```python
from build123d import *

# Parameters (mm, degrees)
F0_W     = 9.525
F0_H     = 18.034
F0_R     = 2.159
F1_DEPTH = 3.175


with BuildPart() as f1:
    # F0 (on Top) → F1 (new body)
    with BuildSketch(Plane.XY):
        with Locations((4.7625, -9.017)):
            Rectangle(F0_W, F0_H)
        with Locations((4.7625, -2.54)):
            Circle(F0_R, mode=Mode.SUBTRACT)
        Polygon((0, -18.034), (0, 0), (-2.54, 0), (-2.54, -21.59), (0, -21.59), align=None)
        Polygon((12.065, 0), (9.525, 0), (9.525, -18.034), (9.525, -21.59), (12.065, -21.59), align=None)
        Polygon((-2.54, 0), (0, 0), (9.525, 0), (12.065, 0), (12.065, 2.54), (-2.54, 2.54), align=None)
        Polygon((9.525, -21.59), (0, -21.59), (-2.54, -21.59), (-2.54, -24.13), (12.065, -24.13), (12.065, -21.59), align=None)
    extrude(amount=F1_DEPTH)


solid = f1.part
```
Geometry check sheet. Reference: the model listing, model coordinates, mm. A direction names the side the tool comes from. Give positions to 0.01 mm unless a question says otherwise; leave off trailing zeros. Order: outer loops, then holes, each group sorted by start corner. A loop starts at its lowest first (then second) coordinate and runs counter-clockwise, first axis right, second up.
1. Section check C-C, the plane z = 1.95. Enter the section's corners in (x, y) (1 decimal).
2. Section check B-B, the plane y = -2.54. Enter the section's corners in (x, z) (1 decimal).
3. Section check A-A, the plane x = 0.75. Enter the section's corners in (y, z) (3 decimals), and give its area (3 significant figures).
4. Thickness scan on L1, parallel to Y at x = 0.25, z = 3; L2, parallel to Y at x = 4.5, z = 0.4; L3, parallel to X at y = -21.5, z = 0.3 (3 decimals). Record the ranges inside material, lowest first.
5. Release check for a two-part mould opening along Y. For faces 1 (the face through (5, -11, 0)), 2 (the face through (5, -21.59, 2)), 3 (the face through (5, 2.54, 2)), 4 (the face through (9.525, -20, 2)) record: pulls with the +Y half, pulls with the -Y half, needs draft (parallel to the pull), parting line crosses it, or undercut.
6. Section check D-D, the plane x = 4.25. Enter the section's corners in (y, z) (3 decimals).
7. Gauge pin test, flat end, axial feed: pin 1 Ø8 at (x, y) = (-1, -9) entering from -Z. Record the tip position at first contact, or that the pin passes through.
8. Access from +Z, -Z, +X, -X, +Y, -Y to the whole of each face (thin tool, end or side, straight path). Record for faces 5 (the face through (12.065, -11, 2)), 6 (the face through (5, -18.034, 2)).
Values follow:
1. outline: (-2.5, -24.1) - (12.1, -24.1) - (12.1, 2.5) - (-2.5, 2.5) - close; hole (0, -21.6) - (9.5, -21.6) - (9.5, -18) - (0, -18) - close; hole circle Ø4.3 at (4.8, -2.5)
2. outline: (-2.5, 0) - (2.6, 0) - (2.6, 3.2) - (-2.5, 3.2) - close; (6.9, 0) - (12.1, 0) - (12.1, 3.2) - (6.9, 3.2) - close
3. outline: (-24.13, 0) - (-21.59, 0) - (-21.59, 3.175) - (-24.13, 3.175) - close; (-18.034, 0) - (2.54, 0) - (2.54, 3.175) - (-18.034, 3.175) - close
3. area: 73.4 mm2
4. L1: y = -24.13 to -21.59, -18.03 to 2.54
4. L2: y = -24.13 to -21.59, -18.03 to -4.68, -0.4 to 2.54
4. L3: x = -2.54 to 0, 9.525 to 12.065
5. face 1: needs draft
5. face 2: undercut
5. face 3: pulls with the +Y half
5. face 4: undercut
6. outline: (-24.13, 0) - (-21.59, 0) - (-21.59, 3.175) - (-24.13, 3.175) - close; (-18.034, 0) - (-4.637, 0) - (-4.637, 3.175) - (-18.034, 3.175) - close; (-0.443, 0) - (2.54, 0) - (2.54, 3.175) - (-0.443, 3.175) - close
7. pin 1: stops at z = 0
8. face 5: +Z, -Z, +X, +Y, -Y
8. face 6: +Z, -Z
